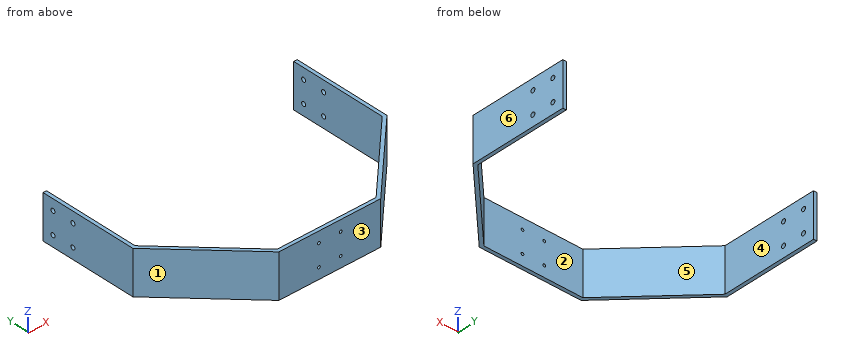
from build123d import *

# Parameters (mm, degrees)
BOSS_EXTRUDE2_DEPTH          = 50.8
F_10_CLEARANCE_HOLE1_D       = 5.1054
F_10_CLEARANCE_HOLE1_DEPTH   = 4.064
F_1_8_0_125_DIAMETER_HOLE1_D = 3.175


with BuildPart() as part:
    # Sketch1 → Boss-Extrude2 (new body)
    with BuildSketch(Plane.XY):
        Polygon((0, 203.2), (0, 88.9), (88.9, 0), (207.772, 0), (296.672, 88.9), (296.672, 203.2), (292.608, 203.2), (292.608, 90.583363917), (206.088636083, 4.064), (90.583363917, 4.064), (4.064, 90.583363917), (4.064, 203.2), align=None)
    extrude(amount=BOSS_EXTRUDE2_DEPTH)

    # #10 Clearance Hole1
    with Locations(Plane(origin=(4.064, 0, 0), x_dir=(0, 0, -1), z_dir=(1, 0, 0))):
        with Locations((-38.1, 190.5), (-12.7, 165.1), (-38.1, 165.1), (-12.7, 190.5)):
            f_10_clearance_hole1 = Hole(F_10_CLEARANCE_HOLE1_D / 2, depth=F_10_CLEARANCE_HOLE1_DEPTH)

    # Mirror1: #10 Clearance Hole1 across plane
    add(f_10_clearance_hole1.mirror(Plane(origin=(148.336, 0, 0), x_dir=(0, 0, 1), z_dir=(1, 0, 0))), mode=Mode.SUBTRACT)

    # 1/8 (0.125) Diameter Hole1 (through all)
    with Locations(Plane(origin=(0, 4.064, 0), x_dir=(1, 0, 0), z_dir=(0, 1, 0))):
        with Locations((135.636, -38.1), (161.036, -12.7), (135.636, -12.7), (161.036, -38.1)):
            Hole(F_1_8_0_125_DIAMETER_HOLE1_D / 2)


solid = part.part
Input: part model. Units: mm. Frame: model coordinates. Face numbers are marked on the shaded views. A direction names the side the tool comes from. Give positions to 0.01 mm unless a question says otherwise; leave off trailing zeros. Loops run counter-clockwise (first coordinate to the right, second up) from the corner with the lowest first, then second, coordinate; pieces in that order, holes last. Notation, with made-up numbers: M -36.5,9 L -26.5,9 A27 cw -26.5,31 Z; hole C 43.5,31 d9. An arc over 180 degrees is marked long. Use CSV: the item, a comma, the result in double quotes.
(1) Section A-A, the plane y = 134. Return loops of the section in (x, z), plus the area to 3 significant figures.
Outcome:
outline,"M 0,0 L 4.06,0 L 4.06,50.8 L 0,50.8 Z; M 292.61,0 L 296.67,0 L 296.67,50.8 L 292.61,50.8 Z"
area,"413 mm²"
(2) Pull-direction query (X, two-part tool) for the marked faces 3, 4, 5 and 6; classes: pulls with the +X half, pulls with the -X half, needs draft (parallel to the pull), parting line crosses it, or undercut.
Outcome:
face 3,"needs draft"
face 4,"undercut"
face 5,"undercut"
face 6,"pulls with the +X half"
(3) Section C-C, the plane x = 112.5. Return loops of the section in (y, z), plus the area to 3 significant figures.
Outcome:
outline,"M 0,0 L 4.06,0 L 4.06,50.8 L 0,50.8 Z"
area,"206 mm²"
(4) Set-up query: the marked faces 1 and 2. Return all of +Z, -Z, +X, -X, +Y, -Y with unobstructed straight access to the full face (end or side cutting, diameter ignored); none if empty.
Outcome:
face 1,"+Z, -Z, -X, -Y"
face 2,"+Z, -Z, +Y"
(5) Section B-B, the plane z = 46. Return loops of the section in (x, y), plus the area to 3 significant figures.
Outcome:
outline,"M 0,88.9 L 88.9,0 L 207.77,0 L 296.67,88.9 L 296.67,203.2 L 292.61,203.2 L 292.61,90.58 L 206.09,4.06 L 90.58,4.06 L 4.06,90.58 L 4.06,203.2 L 0,203.2 Z"
area,"2,410 mm²"
(6) Section D-D, the plane y = 15.5. Return loops of the section in (x, z).
Outcome:
outline,"M 73.4,0 L 79.15,0 L 79.15,50.8 L 73.4,50.8 Z; M 217.52,0 L 223.27,0 L 223.27,50.8 L 217.52,50.8 Z"
(7) Material intervals for L1, parallel to Z at x = 295.3, y = 190.5; L2, parallel to X at y = 139.5, z = 43; L3, parallel to Z at x = 295, y = 190, sorted ascending. Write a range as [from, to].
Outcome:
L1,"z = [0, 10.15], [15.25, 35.55], [40.65, 50.8]"
L2,"x = [0, 4.06], [292.61, 296.67]"
L3,"z = [0, 10.2], [15.2, 35.6], [40.6, 50.8]"
(8) Pin query (flat end, axial travel): P1, Ø10, axis at x = 175.5, z = 43, coming from the +Y side; P2, Ø8, axis at y = 58, z = 45, coming from the +X side; P3, Ø4, axis at x = 241, z = 15.5, coming from the +Y side. Return the tip coordinate at first contact, or that it passes through.
Outcome:
P1,"stops at y = 4.06"
P2,"stops at x = 269.77"
P3,"stops at y = 40.98"
